Can you work these out from the model? Positions are in its coordinate system, mm. A direction names the side the tool comes from. Give positions to 0.01 mm unless a question says otherwise; leave off trailing zeros. Order: outer loops, then holes, each group sorted by start corner. A loop starts at its lowest first (then second) coordinate and runs counter-clockwise, first axis right, second up. Notation, with made-up numbers: (52.5, -11) - (58.5, -11) arc R18 cw to (58.5, -5) - close; hole circle Ø5 at (81.5, 38.25). An arc over 180 degrees is marked (long way). One line per question, with ' | ' between items.
```python
from build123d import *

# Parameters (mm, degrees)
SKETCH1_W           = 60
SKETCH1_H           = 60
BOSS_EXTRUDE1_DEPTH = 15
CUT_EXTRUDE1_DEPTH  = 15
SKETCH8_W           = 15
SKETCH8_H           = 30
BOSS_EXTRUDE2_DEPTH = 160
BOSS_EXTRUDE3_DEPTH = 60
SKETCH10_W          = 8
SKETCH10_H          = 7
BOSS_EXTRUDE4_DEPTH = 20
SKETCH12_R          = 1.9
CUT_EXTRUDE2_DEPTH  = 7
FILLET1_R           = 30
FILLET2_R           = 30
FILLET4_R           = 10
FILLET5_R           = 5


with BuildPart() as part:
    # Sketch1 → Boss-Extrude1 (new body)
    with BuildSketch(Plane(origin=(0, 0, 0), x_dir=(0, 0, -1), z_dir=(1, 0, 0))):
        Rectangle(SKETCH1_W, SKETCH1_H)
    extrude(amount=BOSS_EXTRUDE1_DEPTH)

    # Sketch2 → Cut-Extrude1 (cut)
    with BuildSketch(Plane(origin=(15, 0, 0), x_dir=(0, 0, -1), z_dir=(1, 0, 0))):
        with BuildLine():
            ThreePointArc((2.5, 0), (2.236067977, 1.118033989), (1.5, 2))
            Line((1.5, 2), (-1.5, 2))
            ThreePointArc((-1.5, 2), (-1.118033989, -2.236067977), (2.5, 0))
        make_face()
    extrude(amount=-CUT_EXTRUDE1_DEPTH, mode=Mode.SUBTRACT)

    # Sketch8 → Boss-Extrude2 (add)
    with BuildSketch(Plane.XZ.offset(30)):
        with Locations((7.5, 0)):
            Rectangle(SKETCH8_W, SKETCH8_H)
    extrude(amount=BOSS_EXTRUDE2_DEPTH)

    # Sketch9 → Boss-Extrude3 (add)
    with BuildSketch(Plane.XZ.offset(190)):
        Polygon((0, 0), (0, 30), (15, 30), (15, -30), (0, -30), align=None)
    extrude(amount=BOSS_EXTRUDE3_DEPTH)

    # Sketch10 → Boss-Extrude4 (add)
    with BuildSketch(Plane.ZY):
        with Locations((24.89, -241.5)):
            Rectangle(SKETCH10_W, SKETCH10_H)
        with Locations((-24.89, -241.5)):
            Rectangle(SKETCH10_W, SKETCH10_H)
    extrude(amount=BOSS_EXTRUDE4_DEPTH)

    # Sketch12 → Cut-Extrude2 (cut)
    with BuildSketch(Plane.XZ.offset(245)):
        with Locations(Location((-15.025, 24.89, 0), (0, 0, 270))):
            Circle(SKETCH12_R)
        with Locations(Location((-4.975, 24.89, 0), (0, 0, 270))):
            Circle(SKETCH12_R)
        with Locations(Location((-4.975, -24.89, 0), (0, 0, 270))):
            Circle(SKETCH12_R)
        with Locations(Location((-15.025, -24.89, 0), (0, 0, 270))):
            Circle(SKETCH12_R)
    extrude(amount=-CUT_EXTRUDE2_DEPTH, mode=Mode.SUBTRACT)

    # Fillet1
    # the kernel refuses this fillet: 30 mm, written as the material it takes off along each edge
    with BuildSketch(Plane(origin=(-64.951905284, -30, -30), x_dir=(0, 0, 1), z_dir=(1, 0, 0))) as fillet1_piece_1:
        with BuildLine():
            CenterArc((30, -25.980762114), FILLET1_R, 120, 60)
            Line((0, -25.980762114), (-0.6, -25.980762114))
            Line((-0.6, -25.980762114), (-0.6, 0))
            Line((-0.6, 0), (0, 0.6))
            ThreePointArc((0, 0.6), (7.5, 0.6), (14.7, 0.519615242))
            Line((14.7, 0.519615242), (15, 0))
        make_face()
    extrude(amount=144.903810568, mode=Mode.SUBTRACT)
    with BuildSketch(Plane(origin=(-75, 30, -30), x_dir=(0, 0, 1), z_dir=(1, 0, 0)), Plane(origin=(-75, 30, 30), x_dir=(0, -1, 0), z_dir=(1, 0, 0))) as fillet1_piece_2:
        with BuildLine():
            CenterArc((FILLET1_R, FILLET1_R), FILLET1_R, 180, 90)
            Line((0, FILLET1_R), (-FILLET1_R * 0.02, FILLET1_R))
            Line((-FILLET1_R * 0.02, FILLET1_R), (-FILLET1_R * 0.02, -FILLET1_R * 0.02))
            Line((-FILLET1_R * 0.02, -FILLET1_R * 0.02), (FILLET1_R, -FILLET1_R * 0.02))
            Line((FILLET1_R, -FILLET1_R * 0.02), (FILLET1_R, 0))
        make_face()
    extrude(amount=165, mode=Mode.SUBTRACT)
    with BuildSketch(Plane(origin=(-64.951905284, -30, 30), x_dir=(0, 0, -1), z_dir=(1, 0, 0))) as fillet1_piece_3:
        with BuildLine():
            CenterArc((30, 25.980762114), FILLET1_R, 180, 60)
            Line((0, 25.980762114), (-0.6, 25.980762114))
            Line((-0.6, 25.980762114), (-0.6, 0))
            Line((-0.6, 0), (0, -0.6))
            ThreePointArc((0, -0.6), (7.5, -0.6), (14.7, -0.519615242))
            Line((14.7, -0.519615242), (15, 0))
        make_face()
    extrude(amount=144.903810568, mode=Mode.SUBTRACT)

    # Fillet2
    fillet2_edges = [part.edges().sort_by_distance(p)[0] for p in [
        (7.5, -30, -15),
        (7.5, -30, 15),
    ]]
    fillet(fillet2_edges, radius=FILLET2_R)

    # Fillet4
    fillet4_edges = [part.edges().sort_by_distance(p)[0] for p in [
        (7.5, -190, -15),
        (7.5, -190, 15),
    ]]
    fillet(fillet4_edges, radius=FILLET4_R)

    # Fillet5
    fillet5_edges = [part.edges().sort_by_distance(p)[0] for p in [
        (-20, -241.5, 28.89),
        (-20, -241.5, -28.89),
    ]]
    fillet(fillet5_edges, radius=FILLET5_R)


solid = part.part
```
(1) Imagine slicing it at B-B (y = -96.5). List the corners of the cut face in (x, z) for me.
Answer below:
outline: (0, -15) - (15, -15) - (15, 15) - (0, 15) - close
(2) If we mould it in two halves opening along Y, with no side actions, what happens to faces 1 (the face through (-10, -238, -25)), 2 (the face through (7.6, -186.99, 17.85)), 3 (the face through (-10, -245, 25)), 4 (the face through (15, -108, 0))? For each: released by +Y, released by -Y, zero draft, split by the parting line, or undercut.
Answer below:
face 1: released by +Y | face 2: undercut | face 3: released by -Y | face 4: zero draft
(3) On a 3-axis mill with a long thin cutter (end or side, diameter ignored), from which of +Z, -Z, +X, -X, +Y, -Y can I reach the whole of each face in a straight line? I mean faces 5 (the face through (-10, -242, 20.89)), 6 (the face through (-7, -242, 28.89)), 7 (the face through (-10, -238, 25)), 8 (the face through (8, -190, 28)). Say none if no direction works.
Answer below:
face 5: -X, +Y, -Y | face 6: +Z, -X, +Y, -Y | face 7: +Z, -Z, -X, +Y | face 8: +Z, +X, -X
(4) Imagine slicing it at A-A (x = -10.5). List the corners of the cut face in (y, z) for me, and give its area (3 significant figures).
Answer below:
outline: (-245, -28.89) - (-238, -28.89) - (-238, -20.89) - (-245, -20.89) - close; (-245, 20.89) - (-238, 20.89) - (-238, 28.89) - (-245, 28.89) - close | area: 112 mm^2
(5) If I drill on line 1 (X direction, y = -243, z = 24.89) (3 decimals); line 2 (Y direction, x = 4, z = 0); line 3 (X direction, y = -234.5, z = -23.5), over which ranges is the centre line in solid material (lowest first)?
Answer below:
line 1: -19.899 to -16.925, -13.125 to -6.875, -3.075 to 15 | line 2: -250 to -2.5, 2 to 30 | line 3: 0 to 15
(6) Will these pins go through, and if not, where does the flat tip stop? pin 1 (10 mm diameter, centred on y = -194, z = 12, fed in from -X); pin 2 (12 mm diameter, centred on x = -4.5, z = 2.5, fed in from +Y); pin 3 (2.5 mm diameter, centred on x = 5, z = 28.5, fed in from +Y).
Answer below:
pin 1: x = 0 | pin 2: y = 30 | pin 3: y = 12.55
(7) Imagine slicing it at C-C (z = -10.5). List the corners of the cut face in (x, y) for me, and give its area (3 significant figures).
Answer below:
outline: (0, -250) - (15, -250) - (15, 28.1) - (0, 28.1) - close | area: 4,170 mm^2
